Input: part model. Units: mm. Frame: model coordinates. A direction names the side the tool comes from. Coordinates: 2 decimals unless noted, no trailing zeros. Write each loop counter-clockwise with the first axis right and the second up, starting at its lowest first coordinate (ties: lowest second). Pieces come first, ordered by that corner, then holes.
from build123d import *

# Parameters (mm, degrees)
F0_W     = 20.5
F0_H     = 6
F0_R     = 1
F1_DEPTH = 9
F2_W     = 5.1
F2_H     = 1.8
F3_DEPTH = 20.501
F4_R     = 9
F5_DEPTH = 25


with BuildPart() as f1:
    # F0 (on Top) → F1 (new body)
    with BuildSketch(Plane.XY):
        Rectangle(F0_W, F0_H)
        with Locations((-8.91, 0)):
            Circle(F0_R, mode=Mode.SUBTRACT)
        with Locations((8.91, 0)):
            Circle(F0_R, mode=Mode.SUBTRACT)
    extrude(amount=F1_DEPTH)

    # F2 (on face) → F3 (cut, through all)
    with BuildSketch(Plane.YZ.offset(10.25)):
        with Locations((-0.45, 6.9)):
            Rectangle(F2_W, F2_H)
    extrude(amount=-F3_DEPTH, mode=Mode.SUBTRACT)

    # F4 (on face) → F5 (cut)
    with BuildSketch(Plane(origin=(0, 0, 0), x_dir=(1, 0, 0), z_dir=(0, 0, -1))):
        with Locations((0, 8.41)):
            Circle(F4_R)
    extrude(amount=-F5_DEPTH, mode=Mode.SUBTRACT)


solid = f1.part
Item 1: Section query A-A, the plane x = -8.91. Return loops of the section in (y, z).
Item 2: Pull-direction query (X, two-part tool) for faces 1 (the face through (10.25, 0, 3)), 2 (the face through (9.864, 0.3, 2.958)), 3 (the face through (0, 1, 0)); classes: released by +X, released by -X, zero draft, split by the parting line, or undercut.
Item 3: Section query D-D, the plane y = -0.25. State how many separate pieces and enclosed holes the cut face has, then the cut area to 3 significant figures.
Item 4: Pin query (flat end, axial travel): pin 1 Ø1.4 at (x, z) = (-3, 7) entering from -Y; pin 2 Ø4 at (x, z) = (-0.5, 7.5) entering from -Y; pin 3 Ø1.5 at (x, y) = (-1.5, -0.5) entering from +Z. Return the tip coordinate at first contact, or that it passes through.
Item 5: Access query for faces 4 (the face through (-0.12, 0.59, 2.96)), 5 (the face through (0, 1, 6)). Directions: +Z, -Z, +X, -X, +Y, -Y. A direction counts if a zero-diameter tool reaches every point of the face in a straight line with its end or side. Return the directions, or none.
Item 6: Section query C-C, the plane z = 5.25. Return loops of the section in (x, y), then the cut area to 3 significant figures.
Item 7: Material intervals for line 1 (X direction, y = -0.25, z = 2.25); line 2 (Y direction, x = -8.91, z = 2.1); line 3 (Z direction, x = 3, y = 1), sorted ascending.
Item 8: Section query B-B, the plane y = 1.25. Return loops of the section in (x, z).
The answers:
1. outline: (-3, 0) - (-1, 0) - (-1, 6) - (-3, 6) - close; (-3, 7.8) - (-1, 7.8) - (-1, 9) - (-3, 9) - close; (1, 0) - (3, 0) - (3, 9) - (1, 9) - (1, 7.8) - (2.1, 7.8) - (2.1, 6) - (1, 6) - close
2. face 1: released by +X
2. face 2: undercut
2. face 3: zero draft
3. separate pieces: 8
3. enclosed holes: 0
3. area: 65.0 mm2
4. pin 1: stops at y = 2.1
4. pin 2: stops at y = 0.24
4. pin 3: passes through
5. face 4: +Z, -Z, -Y
5. face 5: +X, -X, -Y
6. outline: (-10.25, -3) - (-7.19, -3) arc R9 cw to (7.19, -3) - (10.25, -3) - (10.25, 3) - (-10.25, 3) - close; hole circle Ø2 at (-8.91, 0); hole circle Ø2 at (8.91, 0)
6. area: 80.6 mm2
7. line 1: x = -10.25 to -9.88, -7.94 to -3.8, 3.8 to 7.94, 9.88 to 10.25
7. line 2: y = -3 to -1, 1 to 3
7. line 3: z = 0 to 6, 7.8 to 9
8. outline: (-10.25, 0) - (10.25, 0) - (10.25, 6) - (-10.25, 6) - close; (-10.25, 7.8) - (10.25, 7.8) - (10.25, 9) - (-10.25, 9) - close
